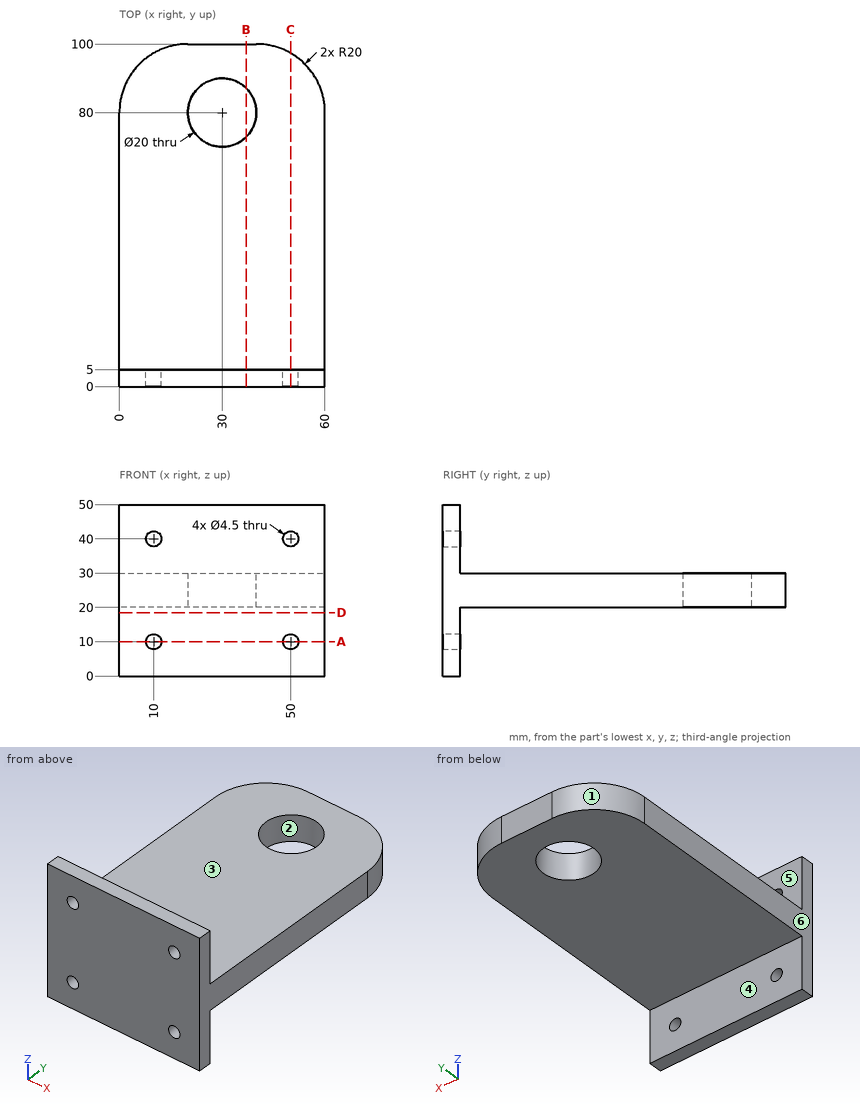
Input: dimensioned drawing with shaded views. Units: mm. Origin: part minimum x, y, z. A direction names the side the tool comes from. Coordinates: 2 decimals unless noted, no trailing zeros. Order: outer loops, then holes, each group sorted by start corner. A loop starts at its lowest first (then second) coordinate and runs counter-clockwise, first axis right, second up.
(1) Section query B-B (x = 37). Return the cut outline in (y, z).
(2) Material intervals for probe 1 along X at (y, z) = (1.8, 40); probe 2 along Y at (x, z) = (30, 24.25); probe 3 along Z at (x, y) = (32.5, 27), sorted ascending.
(3) Draft query along Y for the marked faces 1, 2 and 3. Return one class per face: pulls with the +Y half, pulls with the -Y half, needs draft (parallel to the pull), parting line crosses it, or undercut.
(4) Section query C-C (x = 50). Return the cut outline in (y, z), plus the area to 3 significant figures.
(5) Section query A-A (z = 10). Return the cut outline in (x, y).
(6) Section query D-D (z = 18.5). Return the cut outline in (x, y), plus the area to 3 significant figures.
(7) First-contact query: pin 1 (16 mm diameter, centred on x = 29.5, z = 10, fed in from +Y); pin 2 (16 mm diameter, centred on x = 30, y = 80, fed in from +Z); pin 3 (5 mm diameter, centred on x = 35.5, y = 37.5, fed in from -Z); pin 4 (18 mm diameter, centred on x = 19.5, y = 75.5, fed in from +Z). Flat tips, straight axial feed; report the tip coordinate or a pass-through.
(8) Access query for the marked faces 4, 5 and 6. Directions: +Z, -Z, +X, -X, +Y, -Y. A direction counts if a zero-diameter tool reaches every point of the face in a straight line with its end or side. Return the directions, or none.
Solution:
1. outline: (0, 0) - (5, 0) - (5, 20) - (72.86, 20) - (72.86, 30) - (5, 30) - (5, 50) - (0, 50) - close; (87.14, 20) - (100, 20) - (100, 30) - (87.14, 30) - close
2. probe 1: x = 0 to 7.75, 12.25 to 47.75, 52.25 to 60
2. probe 2: y = 0 to 70, 90 to 100
2. probe 3: z = 20 to 30
3. face 1: pulls with the +Y half
3. face 2: undercut
3. face 3: needs draft
4. outline: (0, 0) - (5, 0) - (5, 7.75) - (0, 7.75) - close; (0, 12.25) - (5, 12.25) - (5, 20) - (97.32, 20) - (97.32, 30) - (5, 30) - (5, 37.75) - (0, 37.75) - close; (0, 42.25) - (5, 42.25) - (5, 50) - (0, 50) - close
4. area: 1,130 mm2
5. outline: (0, 0) - (7.75, 0) - (7.75, 5) - (0, 5) - close; (12.25, 0) - (47.75, 0) - (47.75, 5) - (12.25, 5) - close; (52.25, 0) - (60, 0) - (60, 5) - (52.25, 5) - close
6. outline: (0, 0) - (60, 0) - (60, 5) - (0, 5) - close
6. area: 300 mm2
7. pin 1: stops at y = 5
7. pin 2: passes through
7. pin 3: stops at z = 20
7. pin 4: stops at z = 30
8. face 4: -Z, +X, -X, +Y
8. face 5: +Z, +X, -X, +Y
8. face 6: +Z, -Z, -X, +Y, -Y
